```python
from build123d import *

# Parameters (mm, degrees)
RESSALTO_EXTRUS_O1_DEPTH  = 40
ESBO_O2_OUTSIDE_W         = 151.236
ESBO_O2_OUTSIDE_H         = 155.258
ESBO_O2_OUTSIDE_R         = 13
CORTE_EXTRUS_O1_DEPTH     = 15
CORTE_EXTRUS_O1_DRAFT     = -75
ESBO_O3_OUTSIDE_W         = 151.236
ESBO_O3_OUTSIDE_H         = 155.258
ESBO_O3_OUTSIDE_R         = 13
CORTE_EXTRUS_O2_DEPTH     = 15
CORTE_EXTRUS_O2_DRAFT     = -75
ESBO_O4_R                 = 8.5
RESSALTO_EXTRUS_O2_DEPTH  = 35
FILETE1_R                 = 0.5
FURO_ROSCADO_DE_M61_D     = 5
FURO_ROSCADO_DE_M61_DEPTH = 17
FURO_ROSCADO_DE_M61_TIP   = 1.502151548
ESBO_O7_R                 = 5
CORTE_EXTRUS_O3_DEPTH     = 51.013331556
FILETE2_R                 = 15
FILETE3_R                 = 15


with BuildPart() as part:
    # Esboço1 → Ressalto-extrusão1 (new body)
    with BuildSketch(Plane.XY):
        Polygon((0, 15.011106999), (-13, 7.505553499), (-13, -7.505553499), (0, -15.011106999), (13, -7.505553499), (13, 7.505553499), align=None)
    extrude(amount=RESSALTO_EXTRUS_O1_DEPTH)


with BuildPart() as corte_extrus_o1_tool:
    # Esboço2 outside → Corte-extrusão1 (with draft: the straight prism first)
    with BuildSketch(Plane.XY.offset(40)):
        Rectangle(ESBO_O2_OUTSIDE_W, ESBO_O2_OUTSIDE_H)
        Circle(ESBO_O2_OUTSIDE_R, mode=Mode.SUBTRACT)
    extrude(amount=-CORTE_EXTRUS_O1_DEPTH)
    # Corte-extrusão1: the draft: its side faces are tilted about the plane it starts from
    corte_extrus_o1_sides = [corte_extrus_o1_tool.faces().sort_by_distance(p)[0] for p in [
        (0, -77.629, 32.5),
        (75.618, 0, 32.5),
        (0, 77.629, 32.5),
        (-75.618, 0, 32.5),
        (-13, 0, 32.5),
    ]]
    draft(corte_extrus_o1_sides, Plane.XY.offset(40), CORTE_EXTRUS_O1_DRAFT)


with BuildPart() as part_1:
    add(part.part)

    # Corte-extrusão1: cut by corte_extrus_o1_tool
    add(corte_extrus_o1_tool.part, mode=Mode.SUBTRACT)


with BuildPart() as corte_extrus_o2_tool:
    # Esboço3 outside → Corte-extrusão2 (with draft: the straight prism first)
    with BuildSketch(Plane(origin=(0, 0, 0), x_dir=(-1, 0, 0), z_dir=(0, 0, -1))):
        Rectangle(ESBO_O3_OUTSIDE_W, ESBO_O3_OUTSIDE_H)
        Circle(ESBO_O3_OUTSIDE_R, mode=Mode.SUBTRACT)
    extrude(amount=-CORTE_EXTRUS_O2_DEPTH)
    # Corte-extrusão2: the draft: its side faces are tilted about the plane it starts from
    corte_extrus_o2_sides = [corte_extrus_o2_tool.faces().sort_by_distance(p)[0] for p in [
        (0, -77.629, 7.5),
        (-75.618, 0, 7.5),
        (0, 77.629, 7.5),
        (75.618, 0, 7.5),
        (13, 0, 7.5),
    ]]
    draft(corte_extrus_o2_sides, Plane(origin=(0, 0, 0), x_dir=(-1, 0, 0), z_dir=(0, 0, -1)), CORTE_EXTRUS_O2_DRAFT)


with BuildPart() as part_2:
    add(part_1.part)

    # Corte-extrusão2: cut by corte_extrus_o2_tool
    add(corte_extrus_o2_tool.part, mode=Mode.SUBTRACT)

    # Esboço4 → Ressalto-extrusão2 (add)
    with BuildSketch(Plane(origin=(0, 0, 0), x_dir=(-1, 0, 0), z_dir=(0, 0, -1))):
        with Locations(Location((0, 0, 0), (0, 0, 180))):
            Circle(ESBO_O4_R)
    extrude(amount=RESSALTO_EXTRUS_O2_DEPTH)

    # Filete1
    filete1_edges = [part_2.edges().sort_by_distance(p)[0] for p in [
        (-8.5, 0, -35),
    ]]
    fillet(filete1_edges, radius=FILETE1_R)

    # Furo roscado de M61
    with Locations(Plane(origin=(0, 0, -35), x_dir=(-1, 0, 0), z_dir=(0, 0, -1))):
        with Locations((0, 0)):
            Hole(FURO_ROSCADO_DE_M61_D / 2, depth=FURO_ROSCADO_DE_M61_DEPTH)
            with Locations((0, 0, -(FURO_ROSCADO_DE_M61_DEPTH + FURO_ROSCADO_DE_M61_TIP / 2))):  # 118° drill point
                Cone(0, FURO_ROSCADO_DE_M61_D / 2, FURO_ROSCADO_DE_M61_TIP, mode=Mode.SUBTRACT)

    # Esboço7 → Corte-extrusão3 (cut, through all)
    with BuildSketch(Plane.ZY.offset(13)):
        with Locations(Location((30, 0, 0), (0, 0, 270))):
            Circle(ESBO_O7_R)
    extrude(amount=-CORTE_EXTRUS_O3_DEPTH, mode=Mode.SUBTRACT)

    # Filete2
    # the kernel refuses this fillet: 15 mm, written as the material it takes off along each edge
    with BuildSketch(Plane(origin=(0, 15.011106999, -21.111760598), x_dir=(0.8660254037844415, -0.49999999999999506, 0), z_dir=(0, 0, 1))) as filete2_piece_1:
        with BuildLine():
            CenterArc((FILETE2_R * 0.57735026919, -FILETE2_R), FILETE2_R, 90, 60)
            Line((-FILETE2_R * 0.288675134595, -FILETE2_R * 0.5), (0, 0))
            Line((0, 0), (FILETE2_R * 0.57735026919, 0))
        make_face()
    extrude(amount=82.223521197, mode=Mode.SUBTRACT)

    # Filete3
    # the kernel refuses this fillet: 15 mm, written as the material it takes off along each edge
    with BuildSketch(Plane(origin=(0, -15.011106999, -21.111760598), x_dir=(0.8660254037844344, 0.5000000000000074, 0), z_dir=(0, 0, 1))) as filete3_piece_1:
        with BuildLine():
            CenterArc((FILETE3_R * 0.57735026919, FILETE3_R), FILETE3_R, 210, 60)
            Line((-FILETE3_R * 0.288675134595, FILETE3_R * 0.5), (0, 0))
            Line((0, 0), (FILETE3_R * 0.57735026919, 0))
        make_face()
    extrude(amount=82.223521197, mode=Mode.SUBTRACT)


solid = part_2.part
```
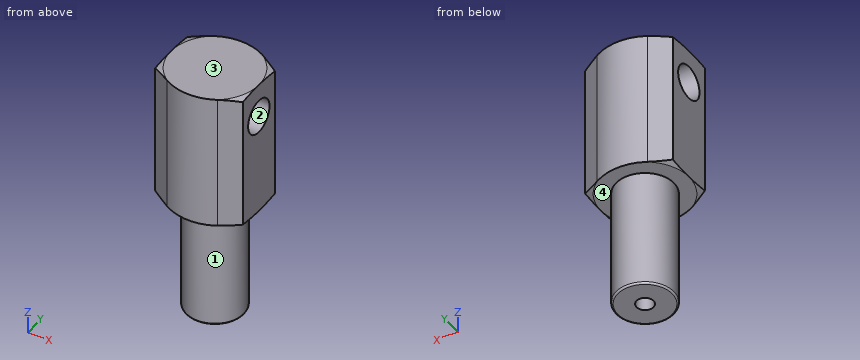
Geometry check sheet. Reference: the model listing, model coordinates, mm. Face numbers are marked on the shaded views. Round coordinates to 2 decimals unless told otherwise and drop trailing zeros. Order: outer loops, then holes, each group sorted by start corner. A loop starts at its lowest first (then second) coordinate and runs counter-clockwise, first axis right, second up. Notation, with made-up numbers: M 6.5,-12.75 L 61.5,-12.75 A9 ccw 61.5,0.25 Z; hole C 3.25,34 d9. An arc over 180 degrees is marked long. Answer as CSV lines item,"result".
1) Sectioned sample at B-B on z = -30. Record the cut outline in (x, y), and give its area (3 significant figures).
Entries:
outline,"C 0,0 d17; hole C 0,0 d5"
area,"207 mm2"
2) Sectioned sample at C-C on z = -9. Record the cut outline in (x, y).
Entries:
outline,"C 0,0 d17"
3) Thickness scan on probe 1 along Z at (x, y) = (4.25, 0); probe 2 along Y at (x, z) = (0, -23.25); probe 3 along Z at (x, y) = (-4.75, -7.75). Record the ranges inside material, lowest first. Write a range as [from, to].
Entries:
probe 1,"[-35, 25], [35, 40]"
probe 2,"[-8.5, -2.5], [2.5, 8.5]"
probe 3,"[0, 40]"
4) Mould release check, pull along Z, two halves, no side actions. Record for the marked faces 1, 2, 3 and 4: +Z half, -Z half, draft (parallel to the pull), parting line (faces both ways), or undercut.
Entries:
face 1,"draft"
face 2,"undercut"
face 3,"+Z half"
face 4,"-Z half"
5) Sectioned sample at A-A on z = 30. Record the cut outline in (x, y).
Entries:
outline,"M -13,-7.51 L -7.5,-10.68 A15 ccw 7.5,-10.68 L 13,-7.51 L 13,-5 L -13,-5 Z; M -13,5 L 13,5 L 13,7.51 L 7.5,10.68 A15 ccw -7.5,10.68 L -13,7.51 Z"
6) Gauge pin test, flat ends, axial feed: pin 1 Ø6 at (x, z) = (-5, -24) entering from +Y; pin 2 Ø4 at (x, z) = (-6, -11) entering from -Y; pin 3 Ø6 at (x, z) = (-10.5, 15) entering from -Y. Record the tip position at first contact, or that the pin passes through.
Entries:
pin 1,"y = 8.26"
pin 2,"y = -7.5"
pin 3,"y = -10.68"
